Source: three-view drawing plus pictorial views. Frame: mm from the lowest corner of the part. A direction names the side the tool comes from. Give positions to 0.01 mm unless a question says otherwise; leave off trailing zeros. Loops run counter-clockwise (first coordinate to the right, second up) from the corner with the lowest first, then second, coordinate; pieces in that order, holes last. Notation, with made-up numbers: (-7.75, -17) - (-1.75, -17) arc R18 cw to (-1.75, -11) - close; hole circle Ø9 at (29.25, 80). An arc over 180 degrees is marked (long way). Answer as a JSON object with one key per item and string values.
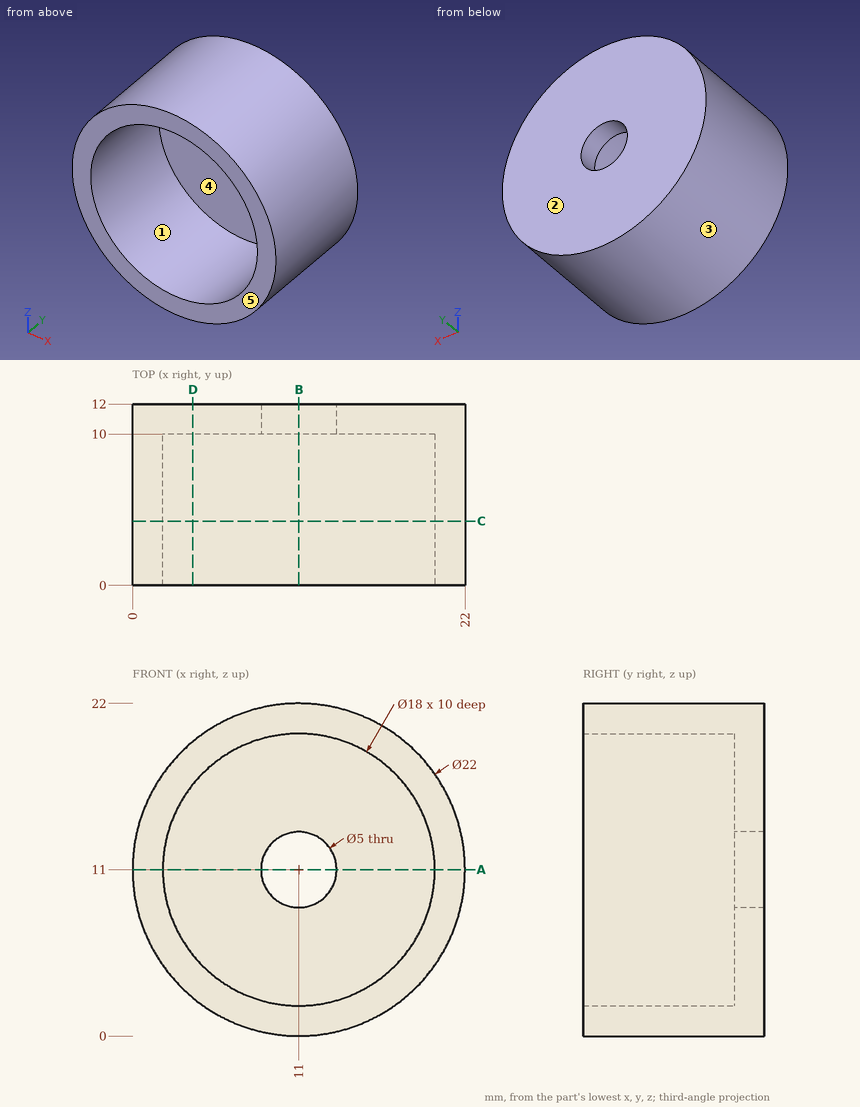
Item 1: Cut plane D-D (x = 4). Return loops of the section in (y, z).
Geometry check:
{"outline": "(0, 2.51) - (12, 2.51) - (12, 19.49) - (0, 19.49) - (0, 16.66) - (10, 16.66) - (10, 5.34) - (0, 5.34) - close"}
Item 2: Cut plane A-A (z = 11). Return loops of the section in (x, y).
Geometry check:
{"outline": "(0, 0) - (2, 0) - (2, 10) - (8.5, 10) - (8.5, 12) - (0, 12) - close; (13.5, 10) - (20, 10) - (20, 0) - (22, 0) - (22, 12) - (13.5, 12) - close"}
Item 3: Access query for the marked faces 4 and 5. Directions: +Z, -Z, +X, -X, +Y, -Y. A direction counts if a zero-diameter tool reaches every point of the face in a straight line with its end or side. Return the directions, or none.
Geometry check:
{"face 4": "-Y", "face 5": "+Z, -Z, +X, -X, -Y"}
Item 4: Mould query, pull axis X, two halves, no side actions, for the marked faces 1, 2 and 3. Classes: released by +X, released by -X, zero draft, split by the parting line, or undercut.
Geometry check:
{"face 1": "undercut", "face 2": "zero draft", "face 3": "split by the parting line"}
Item 5: Material intervals for line 1 (Z direction, x = 11, y = 10.6); line 2 (Z direction, x = 11, y = 3); line 3 (Y direction, x = 6, z = 15), sorted ascending. Write a range as [from, to].
Geometry check:
{"line 1": "z = [0, 8.5], [13.5, 22]", "line 2": "z = [0, 2], [20, 22]", "line 3": "y = [10, 12]"}
Item 6: Cut plane B-B (x = 11). Return loops of the section in (y, z), then the cut area to 3 significant figures.
Geometry check:
{"outline": "(0, 0) - (12, 0) - (12, 8.5) - (10, 8.5) - (10, 2) - (0, 2) - close; (0, 20) - (10, 20) - (10, 13.5) - (12, 13.5) - (12, 22) - (0, 22) - close", "area": "74.0 mm2"}
Item 7: Cut plane C-C (y = 4.25). Return loops of the section in (x, z), then the cut area to 3 significant figures.
Geometry check:
{"outline": "circle Ø22 at (11, 11); hole circle Ø18 at (11, 11)", "area": "126 mm2"}
Item 8: Contact query for flat-ended pins moving along their axis: P1, Ø1, axis at y = 3.5, z = 4.5, coming from the -X side; P2, Ø3, axis at y = 3.5, z = 5, coming from the +X side; P3, Ø9, axis at x = 11.5, z = 11.5, coming from the -Y side. Output: stop coordinate, or through.
Geometry check:
{"P1": "stops at x = 1.78", "P2": "stops at x = 21.04", "P3": "stops at y = 10"}
